For this review, take the finished solid that the model builds, in its own axes (mm). Face numbers are marked on the shaded views. A direction names the side the tool comes from. Give positions to 0.01 mm unless a question says otherwise; leave off trailing zeros. Order: outer loops, then holes, each group sorted by start corner. A loop starts at its lowest first (then second) coordinate and runs counter-clockwise, first axis right, second up. Notation, with made-up numbers: (45, 83) -> (73, 83) arc R15 cw to (73, 91) -> close; hole circle Ø6 at (68, 65.25). An arc over 180 degrees is marked (long way). Return JSON: item names as keys, results as strings. Group by question number.
1) To check wall thickness, follow line 1 along X through (y, z) = (15.5, 0.25); line 2 along X through (y, z) = (4.75, 0). State the ranges of each line that lie inside material, in increasing order.
2) Insertion check: P1, Ø3.5, axis at x = -13, y = 10.5, coming from the -Z side; P2, Ø2, axis at y = 5, z = -2, coming from the +X side; P3, Ø1, axis at x = 1, y = 6, coming from the +Z side. Each pin has a flat end and moves straight along its axis. Give the tip position at first contact, or say it passes through.
3) For the marked faces 4, 5 and 6, list the 3-axis set-ups (+Z, -Z, +X, -X, +Y, -Y) from which the entire face can be reached by the end or side of a thin tool; tool diameter is ignored.
4) Add section A-A (y = 14.75). State how many separate pieces and enclosed holes the cut face has, then the cut area to 3 significant figures.
5) The part is to be moulded in two halves that separate along X. For the marked faces 1, 2 and 3, say which applies: released by +X, released by -X, zero draft, split by the parting line, or undercut.
6) Add section C-C (x = 0). Give the boundary of the cut face in (y, z), then the cut area to 3 significant figures.
7) Add section B-B (y = 3.25). Give the boundary of the cut face in (x, z).
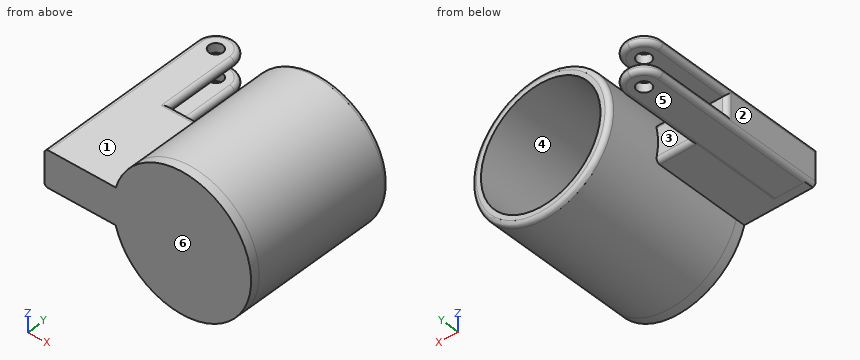
from build123d import *

# Parameters (mm, degrees)
SKETCH1_R                = 7.5
SKETCH1_R_2              = 6.5
BOSS_EXTRUDE2_DEPTH      = 20
SKETCH1_W                = 4
SKETCH1_H                = 1
BOSS_EXTRUDE2_2_DEPTH    = 20
BOSS_EXTRUDE2_3_DEPTH    = 20
BOSS_EXTRUDE3_START      = 1
BOSS_EXTRUDE3_DEPTH      = 1
SKETCH5_W                = 4
SKETCH5_H                = 2
BOSS_EXTRUDE4_DEPTH      = 10
CUT_EXTRUDE5_START       = 16
CUT_EXTRUDE5_OUTLINE_R   = 7.5
CUT_EXTRUDE5_OUTLINE_R_2 = 6.5
CUT_EXTRUDE5_DEPTH       = 4
CUT_EXTRUDE6_DEPTH       = 20
FILLET1_R                = 0.5
FILLET2_R                = 0.5


# Read off the part's stored shape, not the designer's step: Cut-Extrude5
with BuildPart() as part:
    # Sketch1 → Boss-Extrude2 (new body)
    with BuildSketch(Plane(origin=(0, 0, 0), x_dir=(1, 0, 0), z_dir=(0, 1, 0))):
        with Locations(Location((0, 0, 0), (0, 0, 270))):
            Circle(SKETCH1_R)
        with Locations(Location((0, 0, 0), (0, 0, 270))):
            Circle(SKETCH1_R_2, mode=Mode.SUBTRACT)
    extrude(amount=BOSS_EXTRUDE2_DEPTH)



with BuildPart() as body_2:
    # Sketch1 → Boss-Extrude2 2 (new body)
    with BuildSketch(Plane(origin=(0, 0, 0), x_dir=(1, 0, 0), z_dir=(0, 1, 0))):
        with Locations((-13, 1.5)):
            Rectangle(SKETCH1_W, SKETCH1_H)
    extrude(amount=BOSS_EXTRUDE2_2_DEPTH)


with BuildPart() as body_3:
    # Sketch1 → Boss-Extrude2 3 (new body)
    with BuildSketch(Plane(origin=(0, 0, 0), x_dir=(1, 0, 0), z_dir=(0, 1, 0))):
        with Locations((-13, -1.5)):
            Rectangle(SKETCH1_W, SKETCH1_H)
    extrude(amount=BOSS_EXTRUDE2_3_DEPTH)


with BuildPart() as part_1:
    add(part.part)

    add(body_2.part)  # Boss-Extrude3 merges body 2

    add(body_3.part)  # Boss-Extrude3 merges body 3
    # Sketch3 → Boss-Extrude3 (add)
    with BuildSketch(Plane(origin=(0, 0, 0), x_dir=(-1, 0, 0), z_dir=(0, -1, 0)).offset(BOSS_EXTRUDE3_START)):
        with BuildLine():
            Line((15, -2), (7.228416147, -2))
            ThreePointArc((7.228416147, -2), (-7.499972324, 0.020374901), (7.239176027, 1.96069642))
            Line((7.239176027, 1.96069642), (15, 1.96069642))
            Line((15, 1.96069642), (15, -2))
        make_face()
    extrude(amount=-BOSS_EXTRUDE3_DEPTH)

    # Sketch5 → Boss-Extrude4 (add)
    with BuildSketch(Plane(origin=(0, 0, 0), x_dir=(1, 0, 0), z_dir=(0, 1, 0))):
        with BuildLine():
            Line((-11, 1), (-11, -1))
            Line((-11, -1), (-11, -2))
            Line((-11, -2), (-7.228416147, -2))
            ThreePointArc((-7.228416147, -2), (-7.499972324, -0.020374901), (-7.239176027, 1.96069642))
            Line((-7.239176027, 1.96069642), (-11, 1.96069642))
            Line((-11, 1.96069642), (-11, 1))
        make_face()
        with Locations((-13, 0)):
            Rectangle(SKETCH5_W, SKETCH5_H)
    extrude(amount=BOSS_EXTRUDE4_DEPTH)


with BuildPart() as boss_extrude4_kept_piece:
    # of the separate pieces the step leaves, the one the design keeps (boss_extrude4_pieces_kept)
    add(part_1.part.solids().sort_by_distance((0, 0, 7.5))[0])

    # Cut-Extrude5 outline → Cut-Extrude5 (cut)
    with BuildSketch(Plane(origin=(0, 0, 0), x_dir=(1, 0, 0), z_dir=(0, 1, 0)).offset(CUT_EXTRUDE5_START)):
        Circle(CUT_EXTRUDE5_OUTLINE_R)
        Circle(CUT_EXTRUDE5_OUTLINE_R_2, mode=Mode.SUBTRACT)
    extrude(amount=CUT_EXTRUDE5_DEPTH, mode=Mode.SUBTRACT)

    # Sketch7 → Cut-Extrude6 (cut)
    with BuildSketch(Plane.XY.offset(2)):
        with BuildLine():
            ThreePointArc((-12.25, 18), (-13, 18.75), (-13.75, 18))
            Line((-13.75, 18), (-12.25, 18))
        make_face()
        with BuildLine():
            Line((-12.25, 18), (-13.75, 18))
            ThreePointArc((-13.75, 18), (-13, 17.25), (-12.25, 18))
        make_face()
        with BuildLine():
            Line((-11, 20), (-13, 20))
            ThreePointArc((-13, 20), (-11.585786438, 19.414213562), (-11, 18))
            Line((-11, 18), (-11, 20))
        make_face()
        with BuildLine():
            Line((-13, 20), (-15, 20))
            Line((-15, 20), (-15, 18))
            ThreePointArc((-15, 18), (-14.414213562, 19.414213562), (-13, 20))
        make_face()
    extrude(amount=-CUT_EXTRUDE6_DEPTH, mode=Mode.SUBTRACT)

    # Fillet1
    fillet1_edges = [boss_extrude4_kept_piece.edges().sort_by_distance(p)[0] for p in [
        (-15, 9, -2),
        (-11, 9, -2),
        (-15, 14, -1),
        (-11, 14, -1),
        (-11, 14, 1),
        (-15, 14, 1),
        (-11, 14, 2),
        (-15, 8.5, 2),
        (0, 16, -7.5),
        (-13, 20, -2),
        (-13, 20, -1),
        (-13, 20, 1),
        (-13, 20, 2),
    ]]
    fillet(fillet1_edges, radius=FILLET1_R - 0.0001)  # a hair under: the kernel refuses the full size

    # Fillet2
    fillet2_edges = [boss_extrude4_kept_piece.edges().sort_by_distance(p)[0] for p in [
        (-9.272389998, 10, -1.96069642),
        (-15, 10, 0),
        (-9.364158074, 10, 2),
    ]]
    fillet(fillet2_edges, radius=FILLET2_R - 0.0001)  # a hair under: the kernel refuses the full size


solid = boss_extrude4_kept_piece.part
Evaluation:
{
 "1": {"line 1": "-7.5 to -6.5, 6.5 to 7.5", "line 2": "-15 to -6.5, 6.5 to 7.5"},
 "2": {"P1": "z = -2", "P2": "x = 7.43", "P3": "z = 7.48"},
 "3": {"face 4": "+Y", "face 5": "-Z, -X, +Y, -Y", "face 6": "+Z, -Z, +X, -X, -Y"},
 "4": {"separate pieces": "3", "enclosed holes": "1", "area": "51.6 mm^2"},
 "5": {"face 1": "zero draft", "face 2": "released by -X", "face 3": "undercut"},
 "6": {"outline": "(-1, -7.5) -> (15.5, -7.5) arc R0.5 ccw to (16, -7) -> (16, -6.5) -> (0, -6.5) -> (0, 6.5) -> (16, 6.5) -> (16, 7) arc R0.5 ccw to (15.5, 7.5) -> (-1, 7.5) -> close", "area": "46.9 mm^2"},
 "7": {"outline": "(-15, -1.5) arc R0.5 ccw to (-14.5, -2) -> (-11.5, -2) arc R0.5 ccw to (-11.31, -1.96) -> (-7.24, -1.96) arc R7.5 ccw (long way) to (-7.23, 2) -> (-14.5, 2) arc R0.5 ccw to (-15, 1.5) -> close; hole circle Ø13 at (0, 0)"}
}
